Part model, mm, in its own coordinate system. Coordinates: 2 decimals unless noted, no trailing zeros. Order: outer loops, then holes, each group sorted by start corner. A loop starts at its lowest first (then second) coordinate and runs counter-clockwise, first axis right, second up. Notation, with made-up numbers: (-29.5, 73.25) - (2.5, 73.25) arc R8 cw to (2.5, 79.25) - close; hole circle Ø9 at (70.5, 29.25). An arc over 180 degrees is marked (long way). Use a Markdown table: item, result. Add a question column.
1) Saw through at A-A on z = 8. List the corners of the cut face in (x, y).
2) Two-plate mould, pull along X, no slides. Class faces 1 (the face through (31, 2, 0)), 2 (the face through (-19.527, 148.724, 4.93)), 3 (the face through (-1.08, -4.88, 5.07)): +X half, -X half, draft (parallel to the pull), parting line (faces both ways), or undercut.
3) Saw through at B-B on x = -80. List the corners of the cut face in (y, z), then the cut area to 3 significant figures.
4) Drop flat-ended pins along their axis: P1, Ø6.5, axis at x = -140, y = 0, coming from the +Z side; P2, Ø3, axis at y = -25, z = 3.5, coming from the +X side; P3, Ø6, axis at x = 80.5, z = 6.5, coming from the +Y side; P4, Ø5, axis at y = 58, z = 7.5, coming from the +X side. Give the stop position or say it passes through.
5) Wall check: L1, parallel to Y at x = 0, z = 5; L2, parallel to Y at x = 102.5, z = 7.75; L3, parallel to Y at x = 130, z = 8.5. Give the ranges that are in metal, low to high. Write a range as [from, to].
6) Saw through at C-C on y = 74.5. List the corners of the cut face in (x, z).
```python
from build123d import *

# Parameters (mm, degrees)
SKETCH1_R           = 150
BOSS_EXTRUDE1_DEPTH = 10
SKETCH3_R           = 1.5
CUT_EXTRUDE1_DEPTH  = 10
SKETCH5_R           = 1.5
SKETCH5_R_2         = 2
CUT_EXTRUDE2_DEPTH  = 10
SKETCH6_R           = 5
CUT_EXTRUDE8_DEPTH  = 10


with BuildPart() as part:
    # Sketch1 → Boss-Extrude1 (new body)
    with BuildSketch(Plane.XY):
        Circle(SKETCH1_R)
    extrude(amount=BOSS_EXTRUDE1_DEPTH)

    # Sketch3 → Cut-Extrude1 (cut)
    with BuildSketch(Plane.XY.offset(10)):
        with Locations((0, 140)):
            Circle(SKETCH3_R)
    extrude(amount=-CUT_EXTRUDE1_DEPTH, mode=Mode.SUBTRACT)

    # Sketch5 → Cut-Extrude2 (cut)
    with BuildSketch(Plane.XY.offset(10)):
        with Locations((0, -140)):
            Circle(SKETCH5_R)
        with Locations((-140, 0)):
            Circle(SKETCH5_R_2)
        with Locations((140, 0)):
            Circle(SKETCH5_R)
    extrude(amount=-CUT_EXTRUDE2_DEPTH, mode=Mode.SUBTRACT)

    # Sketch6 → Cut-Extrude8 (cut)
    with BuildSketch(Plane.XY.offset(10)):
        Circle(SKETCH6_R)
    extrude(amount=-CUT_EXTRUDE8_DEPTH, mode=Mode.SUBTRACT)


solid = part.part
```
Results are:
| question | item | result |
|---|---|---|
| 1 | outline | circle Ø300 at (0, 0); hole circle Ø4 at (-140, 0); hole circle Ø10 at (0, 0); hole circle Ø3 at (0, -140); hole circle Ø3 at (0, 140); hole circle Ø3 at (140, 0) |
| 2 | face 1 | draft |
| 2 | face 2 | parting line |
| 2 | face 3 | undercut |
| 3 | outline | (-126.89, 0) - (126.89, 0) - (126.89, 10) - (-126.89, 10) - close |
| 3 | area | 2,540 mm2 |
| 4 | P1 | z = 10 |
| 4 | P2 | x = 148.15 |
| 4 | P3 | y = 128.43 |
| 4 | P4 | x = 139.35 |
| 5 | L1 | [-150, -141.5], [-138.5, -5], [5, 138.5], [141.5, 150] |
| 5 | L2 | [-109.52, 109.52] |
| 5 | L3 | [-74.83, 74.83] |
| 6 | outline | (-130.19, 0) - (130.19, 0) - (130.19, 10) - (-130.19, 10) - close |
